The listing builds one solid part. Answer for the finished solid, in the listing's coordinates (mm). Face numbers are marked on the shaded views. Coordinates: 2 decimals unless noted, no trailing zeros. Loops run counter-clockwise (first coordinate to the right, second up) from the corner with the lowest first, then second, coordinate; pieces in that order, holes last. Notation, with made-up numbers: (35, 21.25) - (57, 21.25) arc R9 cw to (57, 31.25) - close; hole circle Ø9 at (2, 9.5). An arc over 180 degrees is marked (long way). Put each result on its own line as item: value.
```python
from build123d import *

# Parameters (mm, degrees)
F0_R     = 10.4166666667
F0_R_2   = 1
F1_DEPTH = 8.3333333333
F2_SIZE2 = 1.0416666667
F2_SIZE  = 4.1666666667
F3_SIZE2 = 4.1666666667
F3_SIZE  = 1.0416666667


with BuildPart() as f1:
    # F0 (on Top) → F1 (new body)
    with BuildSketch(Plane.XY):
        Circle(F0_R)
        Circle(F0_R_2, mode=Mode.SUBTRACT)
    extrude(amount=F1_DEPTH)

    # F2
    f2_edges = [f1.edges().sort_by_distance(p)[0] for p in [
        (-10.416667, 0, 8.333333),
    ]]
    f2_side = f1.faces().sort_by_distance((-10.122039, 0, 8.333333))[0]
    chamfer(f2_edges, length=F2_SIZE, length2=F2_SIZE2, reference=f2_side)

    # F3
    f3_edges = [f1.edges().sort_by_distance(p)[0] for p in [
        (-10.416667, 0, 0),
    ]]
    f3_side = f1.faces().sort_by_distance((-10.416667, 0, 3.645833))[0]
    chamfer(f3_edges, length=F3_SIZE, length2=F3_SIZE2, reference=f3_side)


solid = f1.part
```
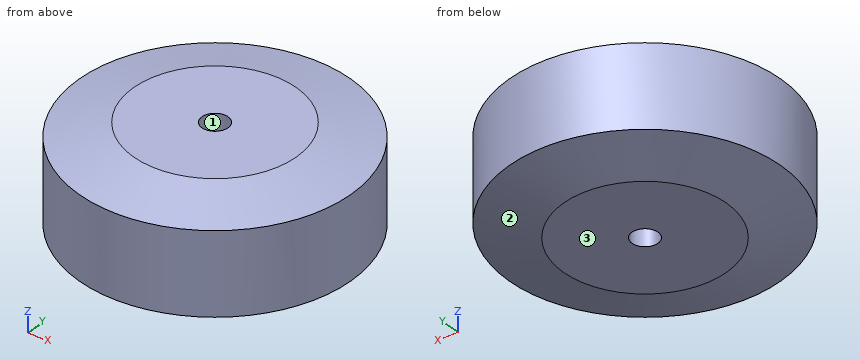
1) Each of these flat-tipped pins is pushed along its axis until it touches: pin 1 (4 mm diameter, centred on x = -7.5, y = 3.5, fed in from +Z); pin 2 (2 mm diameter, centred on x = -2.5, z = 4, fed in from +Y); pin 3 (1.5 mm diameter, centred on y = 7, z = 6, fed in from +X); pin 4 (1.6 mm diameter, centred on x = 0, y = 0, fed in from +Z). Where does it stop, or does it pass through?
Found:
pin 1: stops at z = 8.33
pin 2: stops at y = 10.31
pin 3: stops at x = 8.33
pin 4: passes through
2) Straight lines are drawn through the part: L1, parallel to Y at x = 0, z = 5; L2, parallel to Z at x = -0.75, y = -8.25; L3, parallel to Z at x = -7.5, y = 1. For each, find the intervals that lie inside material, in ascending order. Write a range as [from, to].
Found:
L1: y = [-10.42, -1], [1, 10.42]
L2: z = [0.51, 7.82]
L3: z = [0.33, 8]
3) The part is cut by section C-C (z = 4). Give the vertices of the cut face in (x, y).
Found:
outline: circle Ø20.83 at (0, 0); hole circle Ø2 at (0, 0)
4) The part is cut by section A-A (x = 0). Give the vertices of the cut face in (y, z).
Found:
outline: (-10.42, 1.04) - (-6.25, 0) - (-1, 0) - (-1, 8.33) - (-6.25, 8.33) - (-10.42, 7.29) - close; (1, 0) - (6.25, 0) - (10.42, 1.04) - (10.42, 7.29) - (6.25, 8.33) - (1, 8.33) - close
5) For a pull along Y with two mould halves and no side action, classify the marked faces 1, 2 and 3 as pulls with the +Y half, pulls with the -Y half, needs draft (parallel to the pull), parting line crosses it, or undercut.
Found:
face 1: undercut
face 2: parting line crosses it
face 3: needs draft
